from build123d import *

# Parameters (mm, degrees)
SKETCH_1_R             = 26
SKETCH_1_R_2           = 3
SKETCH_1_R_3           = 5.05
EXTRUDE_1_DEPTH        = 5
FILLET_1_R             = 10
HOLE_WIZARD_M4_1_D     = 3.3
HOLE_WIZARD_M4_1_DEPTH = 10.1
HOLE_WIZARD_M4_1_TIP   = 0.991420021


with BuildPart() as part:
    # 草图1 → 凸台-拉伸1 (new body)
    with BuildSketch(Plane.XY):
        Polygon((-25, 0), (25, 0), (55, 40), (55, 171.5), (26, 201.5), (-26, 201.5), (-55, 171.5), (-55, 40), align=None)
        with Locations((24.438959159, 60)):
            Circle(SKETCH_1_R, mode=Mode.SUBTRACT)
        with Locations((15, 13)):
            Circle(SKETCH_1_R_2, mode=Mode.SUBTRACT)
        with Locations((-15, 13)):
            Circle(SKETCH_1_R_2, mode=Mode.SUBTRACT)
        with Locations((-17.0625, 188.499544236)):
            Circle(SKETCH_1_R_3, mode=Mode.SUBTRACT)
        with Locations((17.0625, 188.499544236)):
            Circle(SKETCH_1_R_3, mode=Mode.SUBTRACT)
        with Locations((-43.875, 122.217270257)):
            Circle(SKETCH_1_R_3, mode=Mode.SUBTRACT)
        with Locations((43.875, 122.217270257)):
            Circle(SKETCH_1_R_3, mode=Mode.SUBTRACT)
    extrude(amount=EXTRUDE_1_DEPTH)

    # 圆角1
    fillet_1_edges = [part.edges().sort_by_distance(p)[0] for p in [
        (-55, 40, 2.5),
        (-55, 171.5, 2.5),
        (-26, 201.5, 2.5),
        (26, 201.5, 2.5),
        (55, 171.5, 2.5),
        (55, 40, 2.5),
        (25, 0, 2.5),
        (-25, 0, 2.5),
    ]]
    fillet(fillet_1_edges, radius=FILLET_1_R)

    # M4 螺纹孔1
    with Locations(Plane(origin=(0, 0, 0), x_dir=(-1, 0, 0), z_dir=(0, 0, -1))):
        with Locations((2.413134666, 89.937895002), (-22.585154319, 90.23038054), (1.705319664, 29.442035657), (-23.292969321, 29.734521195)):
            Hole(HOLE_WIZARD_M4_1_D / 2, depth=HOLE_WIZARD_M4_1_DEPTH)
            with Locations((0, 0, -(HOLE_WIZARD_M4_1_DEPTH + HOLE_WIZARD_M4_1_TIP / 2))):  # 118° drill point
                Cone(0, HOLE_WIZARD_M4_1_D / 2, HOLE_WIZARD_M4_1_TIP, mode=Mode.SUBTRACT)


solid = part.part
Geometry check sheet. Reference: the model listing, model coordinates, mm. Give positions to 0.01 mm unless a question says otherwise; leave off trailing zeros. Order: outer loops, then holes, each group sorted by start corner. A loop starts at its lowest first (then second) coordinate and runs counter-clockwise, first axis right, second up. Notation, with made-up numbers: (8, 37) - (21, 37) arc R4 ccw to (21, 41) - close; hole circle Ø5 at (-21, 75). An arc over 180 degrees is marked (long way). Answer as a JSON object with one key per item and string values.
(1) Cross-section at D-D (z = 3.3). State how many separate pieces and enclosed holes the cut face has, then the cut area to 3 significant figures.
Report:
{"separate pieces": "1", "enclosed holes": "11", "area": "17,500 mm^2"}
(2) Depth check by flat-ended pin: pin 1 Ø2 at (x, z) = (37, 1.5) entering from -Y; pin 2 Ø3.5 at (x, y) = (-15, 13) entering from -Z. Enter the tip coordinate at first touch or a pass-through.
Report:
{"pin 1": "y = 14.67", "pin 2": "through"}
(3) Material ranges on line 1 (X direction, y = 122, z = 0.35); line 2 (X direction, y = 91, z = 1.7); line 3 (Y direction, x = 44, z = 2.25), recorded low to high.
Report:
{"line 1": "-55 to -48.92, -38.83 to 38.83, 48.92 to 55", "line 2": "-55 to -3.68, -1.15 to 21.13, 24.04 to 55", "line 3": "25.33 to 42.87, 77.13 to 117.17, 127.27 to 182.88"}
(4) Cross-section at A-A (y = 60). Record the cut outline in (x, z), then the cut area to 3 significant figures.
Report:
{"outline": "(-55, 0) - (-1.56, 0) - (-1.56, 5) - (-55, 5) - close; (50.44, 0) - (55, 0) - (55, 5) - (50.44, 5) - close", "area": "290 mm^2"}
(5) Cross-section at B-B (x = 9.5). Record the cut outline in (y, z).
Report:
{"outline": "(0, 0) - (38.72, 0) - (38.72, 5) - (0, 5) - close; (81.28, 0) - (201.5, 0) - (201.5, 5) - (81.28, 5) - close"}
(6) Draft check along X on faces 1 (the flat face through (-1, 102, 5)), 2 (the cylindrical face through (-17.4, 11.2, 2.5)), 3 (the cylindrical face through (-25.715, 200.684, 2.535)). Enter one of: released by +X, released by -X, zero draft, split by the parting line, or undercut.
Report:
{"face 1": "zero draft", "face 2": "undercut", "face 3": "released by -X"}
(7) Cross-section at C-C (x = 42). Record the cut outline in (y, z), then the cut area to 3 significant figures.
Report:
{"outline": "(22.67, 0) - (40.83, 0) - (40.83, 5) - (22.67, 5) - close; (79.17, 0) - (117.53, 0) - (117.53, 5) - (79.17, 5) - close; (126.91, 0) - (184.95, 0) - (184.95, 5) - (126.91, 5) - close", "area": "573 mm^2"}
